For this review, take the finished solid that the model builds, in its own axes (mm). Face numbers are marked on the shaded views. Give positions to 0.01 mm unless a question says otherwise; leave off trailing zeros. Write each loop counter-clockwise with the first axis right and the second up, starting at its lowest first coordinate (ties: lowest second). Pieces come first, ordered by that corner, then holes.
Q1. For line 1 (X direction, y = 0, z = -0.25); line 2 (Y direction, x = 0.75, z = 0.3); line 3 (X direction, y = 1, z = 0.8), list the stretches that pass through material, from the lowest coordinate up.
Q2. Mouldability with a two-part tool opening along Y and no side actions: class the marked faces 1, 2 and 3 as released by +Y, released by -Y, zero draft, split by the parting line, or undercut.
Q3. We need section B-B (z = 0.35). Write out the cut boundary in (x, y) (1 decimal), then the cut area to 3 significant figures.
Q4. Insertion check: P1, Ø4.5, axis at x = 0, y = 0, coming from the -Z side; P2, Ø1, axis at x = -1, z = 0, coming from the +Y side. Each pin has a flat end and moves straight along its axis. Give the tip position at first contact, or say it passes through.
Q5. We need section A-A (y = 0). Write out the cut boundary in (x, z).
Q6. We need section C-C (x = -2). Write out the cut boundary in (y, z).
```python
from build123d import *

# Parameters (mm, degrees)
SKETCH1_R          = 1.7525
BASE_EXTRUDE_DEPTH = 1.397


with BuildPart() as part:
    # Sketch1 → Base-Extrude (new body, symmetric)
    with BuildSketch(Plane.XY):
        Polygon((0, 4.54605602), (-3.937, 2.27302801), (-3.937, -2.27302801), (0, -4.54605602), (3.937, -2.27302801), (3.937, 2.27302801), align=None)
        Circle(SKETCH1_R, mode=Mode.SUBTRACT)
    extrude(amount=BASE_EXTRUDE_DEPTH, both=True)

    # Sketch2 → DetailCut (revolve, cut)
    with BuildSketch(Plane(origin=(0, 0, 0), x_dir=(0, 0, -1), z_dir=(1, 0, 0))):
        Polygon((-1.397, 1.7525), (-1.397, 1.8525), (-1.297, 1.7525), align=None)
        with BuildLine():
            Line((-1.397, 4.54605602), (-1.397, 4.04605602))
            ThreePointArc((-1.397, 4.04605602), (-1.250553391, 4.39960941), (-0.897, 4.54605602))
            Line((-0.897, 4.54605602), (-1.397, 4.54605602))
        make_face()
        with BuildLine():
            Line((1.397, 4.54605602), (0.897, 4.54605602))
            ThreePointArc((0.897, 4.54605602), (1.250553391, 4.39960941), (1.397, 4.04605602))
            Line((1.397, 4.04605602), (1.397, 4.54605602))
        make_face()
        Polygon((1.297, 1.7525), (1.397, 1.7525), (1.397, 1.8525), align=None)
    revolve(axis=Axis((0, 0, 0), (0, 0, -1)), mode=Mode.SUBTRACT)


solid = part.part
```
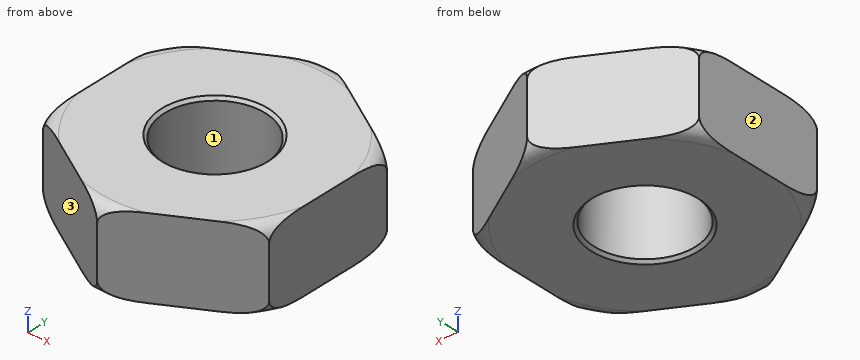
Computed:
1. line 1: x = -3.94 to -1.75, 1.75 to 3.94
1. line 2: y = -4.11 to -1.58, 1.58 to 4.11
1. line 3: x = -3.94 to -1.44, 1.44 to 3.94
2. face 1: undercut
2. face 2: zero draft
2. face 3: released by -Y
3. outline: (-3.9, -2.3) - (0, -4.5) - (3.9, -2.3) - (3.9, 2.3) - (0, 4.5) - (-3.9, 2.3) - close; hole circle Ø3.5 at (0, 0)
3. area: 44.0 mm2
4. P1: stops at z = -1.4
4. P2: stops at y = 4.26
5. outline: (-3.94, -1.4) - (-1.85, -1.4) - (-1.75, -1.3) - (-1.75, 1.3) - (-1.85, 1.4) - (-3.94, 1.4) - close; (1.75, -1.3) - (1.85, -1.4) - (3.94, -1.4) - (3.94, 1.4) - (1.85, 1.4) - (1.75, 1.3) - close
6. outline: (-3.39, -1.4) - (3.39, -1.4) - (3.39, 1.4) - (-3.39, 1.4) - close
